Input: part model. Units: mm. Frame: model coordinates. A direction names the side the tool comes from. Coordinates: 2 decimals unless noted, no trailing zeros. Order: outer loops, then holes, each group sorted by start corner. A loop starts at its lowest first (then second) coordinate and runs counter-clockwise, first axis right, second up. Notation, with made-up numbers: (71.5, 52) -> (123.5, 52) arc R25 cw to (123.5, 80) -> close; hole circle Ø11 at (32, 55.25). An arc over 180 degrees is marked (long way). Write each question's results on one line, items separated by ' | '.
```python
from build123d import *

# Parameters (mm, degrees)
SKETCH_1_R      = 5.5
SKETCH_1_R_2    = 3
EXTRUDE_1_DEPTH = 6
SKETCH_1_3_R    = 3
EXTRUDE_2_DEPTH = 21


with BuildPart() as part:
    # Sketch 1 → Extrude 1 (new body)
    with BuildSketch(Plane.XY):
        Circle(SKETCH_1_R)
        Polygon((4.647669667, 0), (2.323834833, 4.025), (-2.323834833, 4.025), (-4.647669667, 0), (-2.323834833, -4.025), (2.323834833, -4.025), align=None, mode=Mode.SUBTRACT)
        Circle(SKETCH_1_R)
        Circle(SKETCH_1_R_2, mode=Mode.SUBTRACT)
    extrude(amount=EXTRUDE_1_DEPTH)

    # Sketch 1_3 → Extrude 2 (add)
    with BuildSketch(Plane.XY):
        Polygon((4.647669667, 0), (2.323834833, 4.025), (-2.323834833, 4.025), (-4.647669667, 0), (-2.323834833, -4.025), (2.323834833, -4.025), align=None)
        Circle(SKETCH_1_3_R, mode=Mode.SUBTRACT)
    extrude(amount=-EXTRUDE_2_DEPTH)


solid = part.part
```
(1) Cut plane B-B, the plane z = -2. Return loops of the section in (x, y) (3 decimals).
Return value:
outline: (-4.648, 0) -> (-2.324, -4.025) -> (2.324, -4.025) -> (4.648, 0) -> (2.324, 4.025) -> (-2.324, 4.025) -> close; hole circle Ø6 at (0, 0)
(2) Line query: line 1 along Y through (x, z) = (0, 3.65); line 2 along Z through (x, y) = (1.75, 4.75); line 3 along Y through (x, z) = (0, -5.5) (3 decimals). Output: solid intervals per line, ascending. Write a range as from..to.
Return value:
line 1: -5.5..-3, 3..5.5 | line 2: 0..6 | line 3: -4.025..-3, 3..4.025
(3) Pin query (flat end, axial travel): P1, Ø3.5, axis at x = 0.5, z = -12.5, coming from the +Y side (3 decimals); P2, Ø3, axis at y = -2.5, z = -3, coming from the -X side; P3, Ø6, axis at x = 2, z = 1, coming from the +Y side; P4, Ø6, axis at x = 3.5, z = -13.5, coming from the -Y side (3 decimals). Return the tip coordinate at first contact, or that it passes through.
Return value:
P1: y = 4.025 | P2: x = -4.07 | P3: y = 5.5 | P4: y = -4.025
(4) Cut plane D-D, the plane x = -4. Return loops of the section in (y, z), plus the area to 3 significant figures.
Return value:
outline: (-3.77, 0) -> (-1.12, 0) -> (-1.12, -21) -> (1.12, -21) -> (1.12, 0) -> (3.77, 0) -> (3.77, 6) -> (-3.77, 6) -> close | area: 92.4 mm2
(5) Cut plane C-C, the plane y = -0.25. Return loops of the section in (x, z), plus the area to 3 significant figures.
Return value:
outline: (-5.49, 0) -> (-4.5, 0) -> (-4.5, -21) -> (-2.99, -21) -> (-2.99, 6) -> (-5.49, 6) -> close; (2.99, -21) -> (4.5, -21) -> (4.5, 0) -> (5.49, 0) -> (5.49, 6) -> (2.99, 6) -> close | area: 93.6 mm2
(6) Reachability of faces 1 (the face through (-4, -2, 0)), 2 (the face through (3.47, -2.04, -10.35)), 3 (the face through (-3.502, -1.984, -10.353)), 4 (the face through (0, -4.025, -10)), 5 (the face through (0, 4.025, -10)) from +Z, -Z, +X, -X, +Y, -Y: full face, straight path, thin tool, end or side. Return the list, or none.
Return value:
face 1: -Z | face 2: -Z, +X, -Y | face 3: -Z, -X, -Y | face 4: -Z, +X, -X, -Y | face 5: -Z, +X, -X, +Y
(7) Cut plane A-A, the plane x = 0. Return loops of the section in (y, z) (3 decimals), plus the area to 4 significant figures.
Return value:
outline: (-5.5, 0) -> (-4.025, 0) -> (-4.025, -21) -> (-3, -21) -> (-3, 6) -> (-5.5, 6) -> close; (3, -21) -> (4.025, -21) -> (4.025, 0) -> (5.5, 0) -> (5.5, 6) -> (3, 6) -> close | area: 73.05 mm2
